The model under review builds one solid part; all positions refer to its coordinate system, in mm. A direction names the side the tool comes from. Coordinates: 2 decimals unless noted, no trailing zeros. Order: outer loops, then holes, each group sorted by start corner. A loop starts at its lowest first (then second) coordinate and runs counter-clockwise, first axis right, second up.
```python
from build123d import *

# Parameters (mm, degrees)
BOSS_EXTRUDE2_DEPTH = 0.9779
SKETCH5_W           = 0.4953
SKETCH5_H           = 7.366
BOSS_EXTRUDE3_DEPTH = 0.4953
SKETCH6_W           = 0.4953
SKETCH6_H           = 0.4953
BOSS_EXTRUDE4_DEPTH = 4.7625
SKETCH7_W           = 0.4953
SKETCH7_H           = 0.4953
BOSS_EXTRUDE5_DEPTH = 4.7625


with BuildPart() as part:
    # Sketch3 → Revolve1 (revolve)
    with BuildSketch(Plane.XY):
        with BuildLine():
            Line((-2.4638, 5.207), (-2.4638, 0))
            Line((-2.4638, 0), (0, 0))
            Line((0, 0), (0, 7.6708))
            ThreePointArc((0, 7.6708), (-1.742169687, 6.949169687), (-2.4638, 5.207))
        make_face()
    revolve(axis=Axis((0, 0, 0), (0, 1, 0)))

    # Sketch4 → Boss-Extrude2 (add)
    with BuildSketch(Plane.XZ):
        with BuildLine():
            Line((2.55905, 1.421492568), (2.55905, -1.421492568))
            ThreePointArc((2.55905, -1.421492568), (-2.92735, 0), (2.55905, 1.421492568))
        make_face()
    extrude(amount=BOSS_EXTRUDE2_DEPTH)

    # Sketch5 → Boss-Extrude3 (add)
    with BuildSketch(Plane.XY):
        with Locations((-1.30175, -4.6609)):
            Rectangle(SKETCH5_W, SKETCH5_H)
        with Locations((1.30175, -4.6609)):
            Rectangle(SKETCH5_W, SKETCH5_H)
    extrude(amount=BOSS_EXTRUDE3_DEPTH)

    # Sketch6 → Boss-Extrude4 (add)
    with BuildSketch(Plane.XY.offset(0.4953)):
        with Locations((-1.30175, -8.09625)):
            Rectangle(SKETCH6_W, SKETCH6_H)
    extrude(amount=BOSS_EXTRUDE4_DEPTH)

    # Sketch7 → Boss-Extrude5 (add)
    with BuildSketch(Plane.XY.offset(0.4953)):
        with Locations((1.30175, -8.09625)):
            Rectangle(SKETCH7_W, SKETCH7_H)
    extrude(amount=BOSS_EXTRUDE5_DEPTH)


solid = part.part
```
(1) We need section A-A, the plane y = -1.75. Write out the cut boundary in (x, z).
A:
outline: (-1.55, 0) - (-1.05, 0) - (-1.05, 0.5) - (-1.55, 0.5) - close; (1.05, 0) - (1.55, 0) - (1.55, 0.5) - (1.05, 0.5) - close
(2) We need section D-D, the plane y = 4.5. Write out the cut boundary in (x, z), and give its area (3 significant figures).
A:
outline: circle Ø4.93 at (0, 0)
area: 19.1 mm2
(3) For pin 1 Ø0.5 at (x, y) = (-1.5, -4) entering from -Z; pin 2 Ø0.5 at (x, z) = (-1.5, 2.5) entering from +Y; pin 3 Ø1.6 at (x, z) = (1, 1.5) entering from +Y; pin 4 Ø1.6 at (y, z) = (-3, 2.5) entering from -X, all flat-tipped, find the tip position at first contact; note any pin that passes through.
A:
pin 1: stops at z = 0
pin 2: stops at y = 0
pin 3: stops at y = 7.46
pin 4: passes through
(4) We need section C-C, the plane z = 0.75. Write out the cut boundary in (x, y).
A:
outline: (-2.83, -0.98) - (2.56, -0.98) - (2.56, 0) - (2.35, 0) - (2.35, 5.21) arc R2.35 ccw to (-2.35, 5.21) - (-2.35, 0) - (-2.83, 0) - close; (-1.55, -8.34) - (-1.05, -8.34) - (-1.05, -7.85) - (-1.55, -7.85) - close; (1.05, -8.34) - (1.55, -8.34) - (1.55, -7.85) - (1.05, -7.85) - close
(5) Draft analysis for pull direction X (two halves, no side actions). For faces 1 (the face through (-2.925, -0.482, -0.108)), 2 (the face through (1.054, -6, 0.3)), 3 (the face through (1.549, -6, 0.3)), state which applies: released by +X, released by -X, zero draft, split by the parting line, or undercut.
A:
face 1: split by the parting line
face 2: undercut
face 3: released by +X
(6) We need section B-B, the plane x = 0. Write out the cut boundary in (y, z), and give its area (3 significant figures).
A:
outline: (-0.98, -2.93) - (0, -2.93) - (0, -2.46) - (5.21, -2.46) arc R2.46 ccw to (5.21, 2.46) - (0, 2.46) - (0, 2.93) - (-0.98, 2.93) - close
area: 40.9 mm2
(7) Machinability: for faces 4 (the face through (-1.054, -6, 0.3)), 5 (the face through (2.46, 2.57, 0.11)), 6 (the face through (-1.549, -6, 0.3)), which of the approach directions +Z, -Z, +X, -X, +Y, -Y give a long, thin tool a straight path to every point of the face, cutting with its end or side? Answer none if there is none.
A:
face 4: +Z, -Z, -Y
face 5: +Y
face 6: +Z, -Z, -X, -Y
(8) Wall thickness on probe 1 along Y at (x, z) = (-1.15, 2.5); probe 2 along Z at (x, y) = (0, 1.75); probe 3 along Y at (x, z) = (1.1, 4.25): over which ranges is each line inside the solid? List them lowest first.
A:
probe 1: y = -8.34 to -7.85, -0.98 to 0
probe 2: z = -2.46 to 2.46
probe 3: y = -8.34 to -7.85
